Check sheet for the modelled part. Datum: model origin and axes. Units: mm. Coordinates: 2 decimals unless noted, no trailing zeros. Write each loop counter-clockwise with the first axis right and the second up, starting at its lowest first coordinate (ties: lowest second). Pieces come first, ordered by that corner, then holes. Notation, with made-up numbers: M -22,49.5 L -7,49.5 A25 ccw -7,63.5 Z; hole C -0.75,-35.5 d4. An arc over 180 degrees is marked long. Answer as CSV lines item,"result".
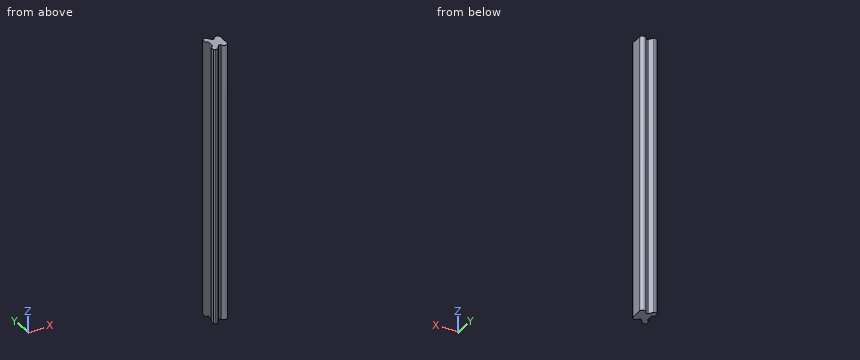
from build123d import *

# Parameters (mm, degrees)
BOSS_EXTRUDE1_DEPTH = 233
FILLET1_R           = 1


with BuildPart() as part:
    # Sketch1 → Boss-Extrude1 (new body)
    with BuildSketch(Plane.XY):
        with BuildLine():
            Line((0, 0), (0, 3.5))
            Line((0, 3.5), (-2, 3.5))
            Line((-2, 3.5), (-2, 8.5))
            Line((-2, 8.5), (1, 8.5))
            Line((1, 8.5), (4, 4.5))
            Line((4, 4.5), (6, 4.5))
            ThreePointArc((6, 4.5), (8.5, 7), (11, 4.5))
            Line((11, 4.5), (11, 0))
            Line((11, 0), (11, -4.5))
            ThreePointArc((11, -4.5), (8.5, -7), (6, -4.5))
            Line((6, -4.5), (4, -4.5))
            Line((4, -4.5), (1, -8.5))
            Line((1, -8.5), (-2, -8.5))
            Line((-2, -8.5), (-2, -3.5))
            Line((-2, -3.5), (0, -3.5))
            Line((0, -3.5), (0, 0))
        make_face()
    extrude(amount=BOSS_EXTRUDE1_DEPTH)

    # Fillet1
    fillet1_edges = [part.edges().sort_by_distance(p)[0] for p in [
        (4, -4.5, 116.5),
        (1, -8.5, 116.5),
        (-2, -8.5, 116.5),
        (-2, -3.5, 116.5),
        (0, -3.5, 116.5),
        (0, 3.5, 116.5),
        (-2, 3.5, 116.5),
        (-2, 8.5, 116.5),
        (1, 8.5, 116.5),
        (4, 4.5, 116.5),
    ]]
    fillet(fillet1_edges, radius=FILLET1_R - 0.0001)  # a hair under: the kernel refuses the full size


solid = part.part
1) Section check B-B, the plane x = 8.5. Record the boundary of the cut face in (y, z), plus the area to 3 significant figures.
Answer key:
outline,"M -7,0 L 7,0 L 7,233 L -7,233 Z"
area,"3,260 mm2"
2) Thickness scan on line 1 along X through (y, z) = (-2, 140.5); line 2 along Y through (x, z) = (5.75, 154); line 3 along Y through (x, z) = (8.25, 110). Record the ranges inside material, lowest first.
Answer key:
line 1,"x = 0 to 11"
line 2,"y = -4.5 to 4.5"
line 3,"y = -6.99 to 6.99"
3) Depth check by flat-ended pin: P1, Ø5, axis at x = 5.5, z = 177, coming from the +Y side; P2, Ø4, axis at y = -0.5, z = 122.5, coming from the -X side; P3, Ø1.5, axis at x = 9.5, z = 106.5, coming from the +Y side; P4, Ø4, axis at x = -0.5, y = -4, coming from the -Z side. Enter the tip coordinate at first touch or a pass-through.
Answer key:
P1,"stops at y = 6.95"
P2,"stops at x = 0"
P3,"stops at y = 6.99"
P4,"stops at z = 0"
